Here's how the part is built. I have some questions about the finished solid (model axes, mm). A direction names the side the tool comes from. Give positions to 0.01 mm unless a question says otherwise; leave off trailing zeros. Write each loop counter-clockwise with the first axis right and the second up, starting at its lowest first coordinate (ties: lowest second). Pieces come first, ordered by that corner, then holes. Notation, with made-up numbers: (69, 15.25) - (116, 15.25) arc R16 ccw to (116, 38.25) - close; hole circle Ø5 at (10.25, 26.5). An arc over 180 degrees is marked (long way). Use one line per item in the form item = value. Start each with the question number.
from build123d import *

# Parameters (mm, degrees)
F0_R     = 82.55
F1_DEPTH = 25.4
F3_DEPTH = 6.35
F4_R     = 1.524


with BuildPart() as f1:
    # F0 (on Front) → F1 (new body)
    with BuildSketch(Plane.XZ):
        Circle(F0_R)
    extrude(amount=F1_DEPTH)

    # F2 (on face) → F3 (cut)
    with BuildSketch(Plane.XZ.offset(25.4)):
        Polygon((49.391409, -49.391409), (69.85, 0), (49.391409, 49.391409), (0, 69.85), (-49.391409, 49.391409), (-69.85, 0), (-49.391409, -49.391409), (0, -69.85), align=None)
    extrude(amount=-F3_DEPTH, mode=Mode.SUBTRACT)

    # F4
    f4_edges = [f1.edges().sort_by_distance(p)[0] for p in [
        (59.620704, -19.05, -24.695704),
        (59.620704, -19.05, 24.695704),
        (24.695704, -19.05, 59.620704),
        (-24.695704, -19.05, 59.620704),
        (-59.620704, -19.05, 24.695704),
        (-59.620704, -19.05, -24.695704),
        (-24.695704, -19.05, -59.620704),
        (24.695704, -19.05, -59.620704),
        (-59.620704, -25.4, 24.695704),
        (-24.695704, -25.4, 59.620704),
        (24.695704, -25.4, 59.620704),
        (59.620704, -25.4, 24.695704),
        (59.620704, -25.4, -24.695704),
        (24.695704, -25.4, -59.620704),
        (-24.695704, -25.4, -59.620704),
        (-59.620704, -25.4, -24.695704),
    ]]
    fillet(f4_edges, radius=F4_R)


solid = f1.part
1. I want a section at A-A, the plane y = -6.5. List the corners of the cut face in (x, z) for me.
2. For faces 4 (the face through (-60.191, -24.965, 24.517)), 5 (the face through (24, -25.4, 62)), which set-ups out of +Z, -Z, +X, -X, +Y, -Y let a thin tool reach every point of the face, with its end or its side?
3. We'd pull the mould along X, two halves only. Please class faces 1 (the face through (-1, 0, 1)), 2 (the face through (-59.898, -24.965, -25.225)), 3 (the face through (-17.895, -12.522, -80.587)): pulls with the +X half, pulls with the -X half, needs draft (parallel to the pull), parting line crosses it, or undercut.
4. For P1, Ø8, axis at x = -30.5, y = -11, coming from the +Z side; P2, Ø1, axis at y = -10.5, z = 5.5, coming from the +X side; P3, Ø12, axis at y = -5, z = -59.5, coming from the +X side, each with a flat end and sliding along its axis, tell me the tip position at first contact or that it passes through.
5. Please list where these lines run through material, in increasing order: line 1 (Y direction, x = 8, z = -45.5); line 2 (X direction, y = -21.25, z = 1.5); line 3 (Z direction, x = 67, y = -15.75).
Result sheet:
q1.outline = circle Ø165.1 at (0, 0)
q2.face_4 = -Y
q2.face_5 = +Z, -Z, +X, -X, -Y
q3.face_1 = needs draft
q3.face_2 = undercut
q3.face_3 = parting line crosses it
q4.P1 = 78.18
q4.P2 = 82.4
q4.P3 = 62.87
q5.line_1 = -19.05 to 0
q5.line_2 = -82.54 to -69.23, 69.23 to 82.54
q5.line_3 = -48.22 to 48.22
